```python
from build123d import *

# Parameters (mm, degrees)
F0_W     = 10
F0_H     = 28
F1_DEPTH = 95
F3_DEPTH = 39.5
F4_W     = 59
F4_H     = 24
F5_DEPTH = 192


with BuildPart() as f1:
    # F0 (on Right) → F1 (new body)
    with BuildSketch(Plane.YZ):
        with Locations((25.561791, -0.421245)):
            Rectangle(F0_W, F0_H)
        Polygon((-29.438209, -29.421245), (-29.438209, -42.421245), (30.561791, -42.421245), (30.561791, -14.421245), (20.561791, -14.421245), align=None)
    extrude(amount=F1_DEPTH)

    # F2 (on face) → F3 (cut)
    with BuildSketch(Plane.XZ.offset(-20.561791)):
        Polygon((95, 13.578755), (57, 13.578755), (95, -14.421245), align=None)
    extrude(amount=-F3_DEPTH, mode=Mode.SUBTRACT)

    # F4 (on Top) → F5 (cut)
    with BuildSketch(Plane.XY):
        with Locations((48.5, -17.497424)):
            Rectangle(F4_W, F4_H)
    extrude(amount=-F5_DEPTH, mode=Mode.SUBTRACT)


solid = f1.part
```
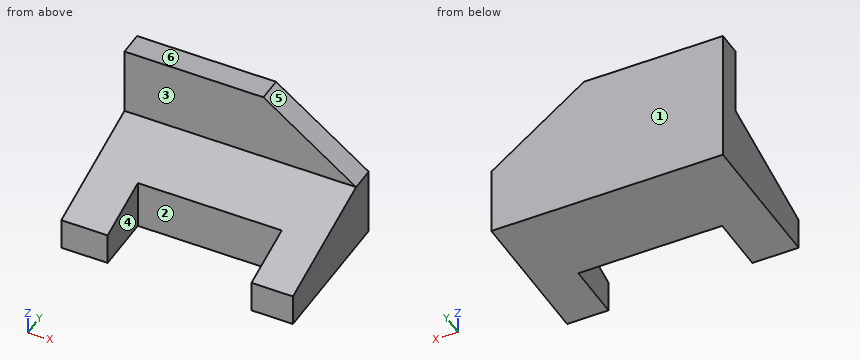
Build history of the part. All positions in model axes, mm. Face numbers are marked on the shaded views. A direction names the side the tool comes from. Give positions to 0.01 mm unless a question says otherwise; leave off trailing zeros. Order: outer loops, then holes, each group sorted by start corner. A loop starts at its lowest first (then second) coordinate and runs counter-clockwise, first axis right, second up. Notation, with made-up numbers: M 28.5,64.25 L 60.5,64.25 A24 cw 60.5,75.25 Z; hole C 86.5,32 d10. An arc over 180 degrees is marked long. Write item = value, one per line. Start each with the question number.
(1) Slice it at B-B on z = -31.5. Write the cut outline in (x, y), plus the area to 3 significant figures.
(2) Which spindle directions (+Z, -Z, +X, -X, +Y, -Y) get a long thin tool onto all of the face, cutting with end or side? Do the marked faces 1, 2 and 3. Say none if no direction does.
(3) Probe L1, parallel to X at y = -16, z = -35.5; L2, parallel to Y at x = 51.5, z = -1; L3, parallel to Y at x = 25, z = -30.5. List the from-to ranges inside material, lowest first. Write a range as [from, to].
(4) Two-plate mould, pull along X, no slides. Class the marked faces 4, 5 and 6: released by +X, released by -X, zero draft, split by the parting line, or undercut.
(5) Slice it at A-A on y = -17. Write the cut outline in (x, z).
(6) Slice it at C-C on x = 16. Write the cut outline in (y, z).
(7) Slice it at D-D on y = -23.5. Write the cut outline in (x, z).
(8) Pin check, flat tips, straight feed: pin 1 Ø8 at (x, y) = (53.5, -9) entering from +Z; pin 2 Ø8.5 at (x, z) = (42, 2) entering from -Y; pin 3 Ø5 at (x, z) = (43.5, -35.5) entering from -Y; pin 4 Ø22 at (y, z) = (-20, -37) entering from -X. Stop position of each tip, or through.
Responses:
q1.outline = M 0,-29.44 L 19,-29.44 L 19,-5.5 L 78,-5.5 L 78,-29.44 L 95,-29.44 L 95,30.56 L 0,30.56 Z
q1.area = 4,290 mm2
q2.face_1 = +Z, -Z, +X, -X, +Y
q2.face_2 = +Z, -Z, -Y
q2.face_3 = +Z, +X, -X, -Y
q3.L1 = [0, 19], [78, 95]
q3.L2 = [20.56, 30.56]
q3.L3 = [-5.5, 30.56]
q4.face_4 = undercut
q4.face_5 = released by +X
q4.face_6 = zero draft
q5.outline = M 0,-42.42 L 19,-42.42 L 19,-25.69 L 0,-25.69 Z; M 78,-42.42 L 95,-42.42 L 95,-25.69 L 78,-25.69 Z
q6.outline = M -29.44,-42.42 L 30.56,-42.42 L 30.56,13.58 L 20.56,13.58 L 20.56,-14.42 L -29.44,-29.42 Z
q7.outline = M 0,-42.42 L 19,-42.42 L 19,-27.64 L 0,-27.64 Z; M 78,-42.42 L 95,-42.42 L 95,-27.64 L 78,-27.64 Z
q8.pin_1 = -22.09
q8.pin_2 = 20.56
q8.pin_3 = -5.5
q8.pin_4 = 0
